Geometry check sheet. Reference: the model listing, model coordinates, mm. Face numbers are marked on the shaded views. A direction names the side the tool comes from. Give positions to 0.01 mm unless a question says otherwise; leave off trailing zeros. Write each loop counter-clockwise with the first axis right and the second up, starting at its lowest first coordinate (ties: lowest second). Pieces come first, ordered by that corner, then holes. Notation, with made-up numbers: (70.5, 71) -> (88.5, 71) arc R17 cw to (88.5, 93) -> close; hole circle Ø8 at (35, -24). An arc over 180 degrees is marked (long way). One line per item, written item: value.
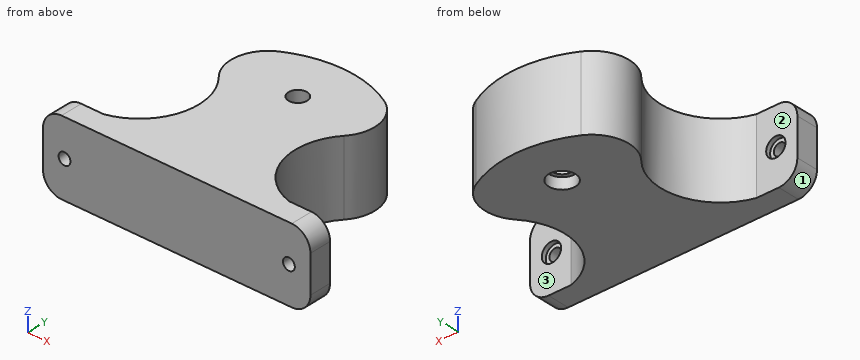
from build123d import *

# Parameters (mm, degrees)
F1_DEPTH = 20
F2_R     = 10
F3_R     = 1.599869
F4_DEPTH = 25
F5_R     = 5
F6_DEPTH = 3
F3_R_2   = 2.6
F7_DEPTH = 1.2


with BuildPart() as f1:
    # F0 (on Top) → F1 (new body)
    with BuildSketch(Plane.XY):
        with BuildLine():
            Line((25, 15.5), (3.6, 15.5))
            ThreePointArc((3.6, 15.5), (0, 11.9), (-3.6, 15.5))
            Line((-3.6, 15.5), (-25, 15.5))
            ThreePointArc((-25, 15.5), (-12.968627, 0), (-25, -15.5))
            Line((-25, -15.5), (25, -15.5))
            ThreePointArc((25, -15.5), (12.968627, 0), (25, 15.5))
        make_face()
        with BuildLine():
            ThreePointArc((-2.5, 15.5), (0, 18), (2.5, 15.5))
            Line((2.5, 15.5), (3.6, 15.5))
            ThreePointArc((3.6, 15.5), (0, 19.1), (-3.6, 15.5))
            Line((-3.6, 15.5), (-2.5, 15.5))
        make_face()
        with BuildLine():
            ThreePointArc((-20.07486, -21.5), (-22.736221, -18.663179), (-25, -15.5))
            Line((-25, -15.5), (-36, -15.5))
            Line((-36, -15.5), (-36, -21.5))
            Line((-36, -21.5), (-20.07486, -21.5))
        make_face()
        with BuildLine():
            ThreePointArc((20.07486, -21.5), (22.736221, -18.663179), (25, -15.5))
            Line((25, -15.5), (-25, -15.5))
            ThreePointArc((-25, -15.5), (-22.736221, -18.663179), (-20.07486, -21.5))
            Line((-20.07486, -21.5), (20.07486, -21.5))
        make_face()
        with BuildLine():
            Line((36, -15.5), (25, -15.5))
            ThreePointArc((25, -15.5), (22.736221, -18.663179), (20.07486, -21.5))
            Line((20.07486, -21.5), (36, -21.5))
            Line((36, -21.5), (36, -15.5))
        make_face()
        with BuildLine():
            ThreePointArc((-3.6, 15.5), (0, 19.1), (3.6, 15.5))
            Line((3.6, 15.5), (25, 15.5))
            ThreePointArc((25, 15.5), (0, 29.415132), (-25, 15.5))
            Line((-25, 15.5), (-3.6, 15.5))
        make_face()
        with BuildLine():
            Line((3.6, 15.5), (2.5, 15.5))
            ThreePointArc((2.5, 15.5), (0, 13), (-2.5, 15.5))
            Line((-2.5, 15.5), (-3.6, 15.5))
            ThreePointArc((-3.6, 15.5), (0, 11.9), (3.6, 15.5))
        make_face()
    extrude(amount=F1_DEPTH)

    # F2
    f2_edges = [f1.edges().sort_by_distance(p)[0] for p in [
        (25, 15.5, 10),
        (-25, 15.5, 10),
    ]]
    fillet(f2_edges, radius=F2_R)

    # F3 (on face) → F4 (cut)
    with BuildSketch(Plane(origin=(0, -15.5, 0), x_dir=(-1, 0, 0), z_dir=(0, 1, 0))):
        with Locations((30.207418, 10)):
            Circle(F3_R)
        with Locations((-30.207418, 10)):
            Circle(F3_R)
    extrude(amount=-F4_DEPTH, mode=Mode.SUBTRACT)

    # F5
    f5_edges = [f1.edges().sort_by_distance(p)[0] for p in [
        (-36, -18.5, 20),
        (36, -18.5, 20),
        (36, -18.5, 0),
        (-36, -18.5, 0),
    ]]
    fillet(f5_edges, radius=F5_R)

    # F0 (on Top) → F6 (cut)
    with BuildSketch(Plane.XY):
        with BuildLine():
            ThreePointArc((-2.5, 15.5), (0, 18), (2.5, 15.5))
            Line((2.5, 15.5), (3.6, 15.5))
            ThreePointArc((3.6, 15.5), (0, 19.1), (-3.6, 15.5))
            Line((-3.6, 15.5), (-2.5, 15.5))
        make_face()
        with BuildLine():
            Line((3.6, 15.5), (2.5, 15.5))
            ThreePointArc((2.5, 15.5), (0, 13), (-2.5, 15.5))
            Line((-2.5, 15.5), (-3.6, 15.5))
            ThreePointArc((-3.6, 15.5), (0, 11.9), (3.6, 15.5))
        make_face()
    extrude(amount=F6_DEPTH, mode=Mode.SUBTRACT)

    # F3 (on face) → F7 (cut)
    with BuildSketch(Plane(origin=(0, -15.5, 0), x_dir=(-1, 0, 0), z_dir=(0, 1, 0))):
        with Locations((-30.207418, 10)):
            Circle(F3_R_2)
        with Locations((-30.207418, 10)):
            Circle(F3_R, mode=Mode.SUBTRACT)
        with Locations((30.207418, 10)):
            Circle(F3_R_2)
        with Locations((30.207418, 10)):
            Circle(F3_R, mode=Mode.SUBTRACT)
    extrude(amount=-F7_DEPTH, mode=Mode.SUBTRACT)


solid = f1.part
1) Sectioned sample at A-A on x = 0. Record the cut outline in (y, z), plus the area to 3 significant figures.
Verdict:
outline: (-21.5, 0) -> (11.9, 0) -> (11.9, 3) -> (13, 3) -> (13, 20) -> (-21.5, 20) -> close; (18, 3) -> (19.1, 3) -> (19.1, 0) -> (29.42, 0) -> (29.42, 20) -> (18, 20) -> close
area: 912 mm^2
2) Depth check by flat-ended pin: pin 1 Ø1.5 at (x, z) = (-15, 18) entering from +Y; pin 2 Ø9 at (x, z) = (-33, 5.5) entering from +Y; pin 3 Ø10 at (y, z) = (0.5, 8.5) entering from -X. Enter the tip coordinate at first touch or a pass-through.
Verdict:
pin 1: y = 25.73
pin 2: y = -15.5
pin 3: x = -13.94
3) Sectioned sample at B-B on y = -8. Record the cut outline in (x, z), plus the area to 3 significant figures.
Verdict:
outline: (-15.11, 0) -> (15.11, 0) -> (15.11, 20) -> (-15.11, 20) -> close
area: 604 mm^2
4) Scan lines: probe 1 along Y at (x, z) = (-28.5, 8); probe 2 along X at (y, z) = (0.5, 4.25); probe 3 along Y at (x, z) = (-17.5, 2.25). Record each from-to range of solid material in increasing order.
Verdict:
probe 1: -21.5 to -15.5
probe 2: -12.98 to 12.98
probe 3: -21.5 to -11.16, 11.27 to 22.79
5) Tool access check on the marked faces 1, 2 and 3. Record the directions out of +Z, -Z, +X, -X, +Y, -Y that give a thin tool (end or side, any length) a straight path to the whole face; none if there is none.
Verdict:
face 1: -Z, -X, +Y, -Y
face 2: +Z, -Z, -X, +Y
face 3: +Z, -Z, +X, +Y
6) Sectioned sample at C-C on y = -2. Record the cut outline in (x, z), plus the area to 3 significant figures.
Verdict:
outline: (-13.09, 0) -> (13.09, 0) -> (13.09, 20) -> (-13.09, 20) -> close
area: 524 mm^2
